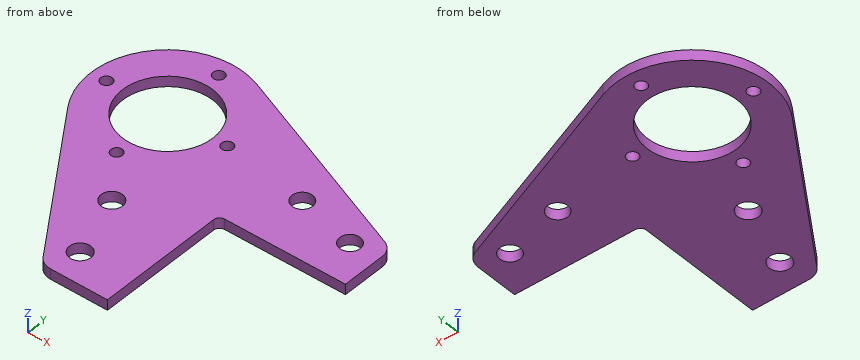
```python
from build123d import *

# Parameters (mm, degrees)
SKETCH1_R          = 1.75
SKETCH1_R_2        = 13.8
BASE_FLANGE1_DEPTH = 3.175
SKETCH6_R          = 3.15
SKETCH6_R_2        = 3.282457618
CUT_EXTRUDE1_DEPTH = 128.736584442


# Sheet-metal steps are written as plain solids
with BuildPart() as part:
    # Sketch1 → Base-Flange1 (new body)
    with BuildSketch(Plane.XY):
        with BuildLine():
            Line((38.970667364, 0.451979476), (56.476339415, 0.364231306))
            Line((56.476339415, 0.364231306), (56.476339415, 38.864663006))
            ThreePointArc((56.476339415, 38.864663006), (57.009920449, 40.134796597), (58.285339291, 40.655617905))
            Line((58.285339291, 40.655617905), (95.285804475, 40.655617905))
            Line((95.285804475, 40.655617905), (95.285804475, 53.835620703))
            ThreePointArc((95.285804475, 53.835620703), (94.475239571, 56.617857644), (92.257476371, 58.483168407))
            Line((92.257476371, 58.483168407), (32.202639785, 83.238911906))
            ThreePointArc((32.202639785, 83.238911906), (5.007775741, 76.331219775), (3.813808252, 48.29818065))
            Line((3.813808252, 48.29818065), (34.861096289, 2.640368074))
            ThreePointArc((34.861096289, 2.640368074), (36.645617305, 1.038644509), (38.970667364, 0.451979476))
        make_face()
        with Locations((23.246582606, 43.012689186)):
            Circle(SKETCH1_R, mode=Mode.SUBTRACT)
        with Locations((4.493399578, 61.512456777)):
            Circle(SKETCH1_R, mode=Mode.SUBTRACT)
        with Locations((23.246582606, 80.012224369)):
            Circle(SKETCH1_R, mode=Mode.SUBTRACT)
        with Locations((41.492934761, 61.512456777)):
            Circle(SKETCH1_R, mode=Mode.SUBTRACT)
        with Locations((23.246582606, 61.512456777)):
            Circle(SKETCH1_R_2, mode=Mode.SUBTRACT)
    extrude(amount=-BASE_FLANGE1_DEPTH)

    # Sketch6 → Cut-Extrude1 (cut, through all)
    with BuildSketch(Plane.XY):
        with Locations((86.341786245, 52.887725453)):
            Circle(SKETCH6_R)
        with Locations((40.269797133, 9.667877899)):
            Circle(SKETCH6_R_2)
        with Locations((33.701172349, 28.884316382)):
            Circle(SKETCH6_R_2)
        with Locations((67.843667948, 57.502749994)):
            Circle(SKETCH6_R)
    extrude(amount=-CUT_EXTRUDE1_DEPTH, mode=Mode.SUBTRACT)


solid = part.part
```
Can you work these out from the model? Positions are in its coordinate system, mm. Coordinates: 2 decimals unless noted, no trailing zeros. Order: outer loops, then holes, each group sorted by start corner. A loop starts at its lowest first (then second) coordinate and runs counter-clockwise, first axis right, second up.
1. I need wall thicknesses on line 1 (Y direction, x = 35, z = -1.4); line 2 (X direction, y = 61.5, z = -2.6); line 3 (X direction, y = 53, z = -2.45). Which ranges of each line are inside material? Lowest first, please.
2. If we section it at C-C (z = -1.6): Give the number of separate pieces and of enclosed holes in the cut face, then the cut area to 3 significant figures.
3. I'm going to push flat-ended pins straight in: pin 1 (1 mm diameter, centred on x = 38, z = -1, fed in from +Y); pin 2 (1 mm diameter, centred on y = 23.5, z = -2, fed in from +X); pin 3 (1.5 mm diameter, centred on x = 42.5, z = -2, fed in from +Y). Where does each tip first touch, or does it pass through?
4. If we section it at D-D (y = 22): Please give me the cut outline in (x, z) (3 decimals).
5. If we section it at B-B (y = 70.5): Please give me the cut outline in (x, z) (3 decimals), then the cut area to 3 significant figures.
6. If we section it at A-A (x = 68): Please give me the cut outline in (y, z) (3 decimals), then the cut area to 3 significant figures.
Entries:
1. line 1: y = 2.45 to 25.87, 31.9 to 54.28, 68.74 to 82.09
1. line 2: x = -0.25 to 2.74, 6.24 to 9.45, 37.05 to 39.74, 43.24 to 84.94
1. line 3: x = 1.34 to 12.38, 34.11 to 83.19, 89.49 to 95.29
2. separate pieces: 1
2. enclosed holes: 9
2. area: 3,700 mm2
3. pin 1: stops at y = 81.06
3. pin 2: stops at x = 56.48
3. pin 3: stops at y = 79.3
4. outline: (21.697, -3.175) - (56.476, -3.175) - (56.476, 0) - (21.697, 0) - close
5. outline: (1.533, -3.175) - (12.775, -3.175) - (12.775, 0) - (1.533, 0) - close; (33.719, -3.175) - (63.106, -3.175) - (63.106, 0) - (33.719, 0) - close
5. area: 129 mm2
6. outline: (40.656, -3.175) - (54.357, -3.175) - (54.357, 0) - (40.656, 0) - close; (60.649, -3.175) - (68.483, -3.175) - (68.483, 0) - (60.649, 0) - close
6. area: 68.4 mm2
